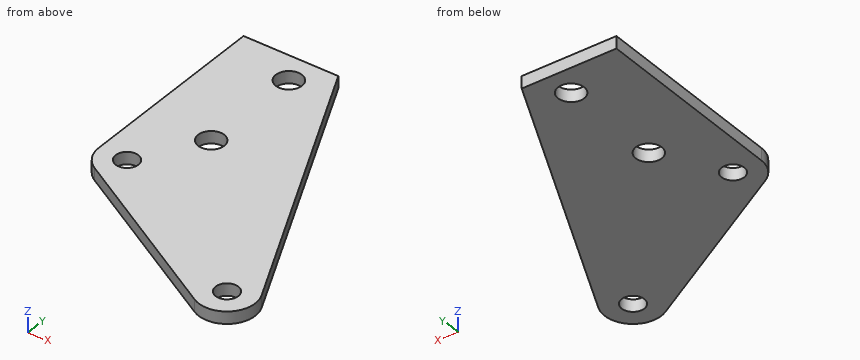
```python
from build123d import *

# Parameters (mm, degrees)
F0_R     = 1.5875
F0_R_2   = 1.8288
F1_DEPTH = 1.70942


with BuildPart() as f1:
    # F0 (on Top) → F1 (new body)
    with BuildSketch(Plane.XY):
        with BuildLine():
            Line((13.24008, 0), (0, 0))
            Line((0, 0), (0, -27.3685))
            ThreePointArc((0, -27.3685), (0.531712, -29.352875), (1.984375, -30.805538))
            Line((1.984375, -30.805538), (26.374369, -44.887108))
            ThreePointArc((26.374369, -44.887108), (31.045093, -44.371457), (31.949778, -39.760262))
            Line((31.949778, -39.760262), (13.24008, 0))
        make_face()
        with Locations((3.96875, -27.3685)):
            Circle(F0_R, mode=Mode.SUBTRACT)
        with Locations((28.358744, -41.45007)):
            Circle(F0_R, mode=Mode.SUBTRACT)
        with Locations((9.27133, -18.63725)):
            Circle(F0_R_2, mode=Mode.SUBTRACT)
        with Locations((9.27133, -3.96875)):
            Circle(F0_R_2, mode=Mode.SUBTRACT)
    extrude(amount=F1_DEPTH)


solid = f1.part
```
Work out the finished part from the listing and answer in its coordinate system (mm). Give positions to 0.01 mm unless a question says otherwise; leave off trailing zeros. Loops run counter-clockwise (first coordinate to the right, second up) from the corner with the lowest first, then second, coordinate; pieces in that order, holes last. Notation, with made-up numbers: M 33,81 L 60,81 A13 ccw 60,90 Z; hole C 76.25,3.5 d5. An arc over 180 degrees is marked long. One line per item, written item: value. Start each with the question number.
1. Find section B-B (x = 28). Give the vertices of the cut face in (y, z).
2. Find section D-D (y = -7.5). Give the vertices of the cut face in (x, z), and give its area (3 significant figures).
3. Each of these flat-tipped pins is pushed along its axis until it touches: P1, Ø3.5, axis at x = 9.27, y = -18.64, coming from the +Z side; P2, Ø1, axis at y = -11.5, z = 0, coming from the +X side. Where does it stop, or does it pass through?
4. Find the intervals of material crossed by probe 1 along X at (y, z) = (-3, 1.3); probe 2 along Y at (x, z) = (27, 1.2); probe 3 along Y at (x, z) = (19, 0.95), in increasing order.
5. Find section A-A (y = -17.5). Give the vertices of the cut face in (x, z), and give its area (3 significant figures).
6. Find section C-C (z = 1.1). Give the vertices of the cut face in (x, y) (1 decimal), and give its area (3 significant figures).
Reported:
1. outline: M -45.4,0 L -43,0 L -43,1.71 L -45.4,1.71 Z; M -39.9,0 L -31.37,0 L -31.37,1.71 L -39.9,1.71 Z
2. outline: M 0,0 L 16.77,0 L 16.77,1.71 L 0,1.71 Z
2. area: 28.7 mm²
3. P1: passes through
3. P2: stops at x = 18.89
4. probe 1: x = 0 to 7.72, 10.82 to 14.65
4. probe 2: y = -45.18 to -42.27, -40.63 to -29.24
4. probe 3: y = -40.63 to -12.24
5. outline: M 0,0 L 7.84,0 L 7.84,1.71 L 0,1.71 Z; M 10.7,0 L 21.47,0 L 21.47,1.71 L 10.7,1.71 Z
5. area: 31.8 mm²
6. outline: M 0,-27.4 A4 ccw 2,-30.8 L 26.4,-44.9 A4 ccw 31.9,-39.8 L 13.2,0 L 0,0 Z; hole C 4,-27.4 d3.2; hole C 9.3,-18.6 d3.7; hole C 9.3,-4 d3.7; hole C 28.4,-41.5 d3.2
6. area: 825 mm²
